Design review of the part built by this model. Coordinates are the model's own, in mm. A direction names the side the tool comes from. Give positions to 0.01 mm unless a question says otherwise; leave off trailing zeros. Order: outer loops, then holes, each group sorted by start corner. A loop starts at its lowest first (then second) coordinate and runs counter-clockwise, first axis right, second up. Notation, with made-up numbers: M 20.25,9.25 L 42.25,9.25 A33 ccw 42.25,37.25 Z; hole C -22,71 d6. An arc over 180 degrees is marked long. Answer as a JSON object with one key per item and string values.
from build123d import *

# Parameters (mm, degrees)
SKETCH1_W             = 152.4
SKETCH1_H             = 19.05
SKETCH1_R             = 4
BOSS_EXTRUDE1_DEPTH   = 25.4
SKETCH3_R             = 25.05
CUT_EXTRUDE1_DEPTH    = 22
M10_CLEARANCE_HOLE1_D = 11
SKETCH11_R            = 2.5
CUT_EXTRUDE2_DEPTH    = 10


with BuildPart() as part:
    # Sketch1 → Boss-Extrude1 (new body)
    with BuildSketch(Plane.XY):
        with Locations((0, -34.525)):
            Rectangle(SKETCH1_W, SKETCH1_H)
        with BuildLine():
            Line((-37.7, -25), (37.7, -25))
            Line((37.7, -25), (37.7, 0))
            ThreePointArc((37.7, 0), (0, 37.7), (-37.7, 0))
            Line((-37.7, 0), (-37.7, -25))
        make_face()
        Circle(SKETCH1_R, mode=Mode.SUBTRACT)
    extrude(amount=BOSS_EXTRUDE1_DEPTH)

    # Sketch3 → Cut-Extrude1 (cut)
    with BuildSketch(Plane.XY.offset(25.4)):
        Circle(SKETCH3_R)
    extrude(amount=-CUT_EXTRUDE1_DEPTH, mode=Mode.SUBTRACT)

    # M10 Clearance Hole1 (through all)
    with Locations(Plane(origin=(0, -25, 0), x_dir=(1, 0, 0), z_dir=(0, 1, 0))):
        with Locations((-57.2, -12.7), (57.2, -12.7)):
            Hole(M10_CLEARANCE_HOLE1_D / 2)

    # Sketch11 → Cut-Extrude2 (cut)
    with BuildSketch(Plane(origin=(0, 0, 0), x_dir=(-1, 0, 0), z_dir=(0, 0, -1))):
        with Locations((5.775120383, 13.84369837)):
            Circle(SKETCH11_R)
        with Locations((-5.705346209, 13.872599779)):
            Circle(SKETCH11_R)
        with Locations((-13.84369837, 5.775120383)):
            Circle(SKETCH11_R)
        with Locations((-13.872599779, -5.705346209)):
            Circle(SKETCH11_R)
        with Locations((-5.775120383, -13.84369837)):
            Circle(SKETCH11_R)
        with Locations((5.705346209, -13.872599779)):
            Circle(SKETCH11_R)
        with Locations((13.84369837, -5.775120383)):
            Circle(SKETCH11_R)
        with Locations((13.872599779, 5.705346209)):
            Circle(SKETCH11_R)
    extrude(amount=-CUT_EXTRUDE2_DEPTH, mode=Mode.SUBTRACT)


solid = part.part
(1) Draft analysis for pull direction Z (two halves, no side actions). For faces 1 (the flat face through (-1, -12, 0)), 2 (the cylindrical face through (-16.257, 6.456, 1.676)), 3 (the cylindrical face through (62.695, -34.658, 12.458)), 4 (the cylindrical face through (-51.705, -34.658, 12.458)), state which applies: +Z half, -Z half, draft (parallel to the pull), parting line (faces both ways), or undercut.
Checked values:
{"face 1": "-Z half", "face 2": "draft", "face 3": "undercut", "face 4": "undercut"}
(2) We need section D-D (x = 57.2). Write out the cut boundary in (y, z), plus the area to 3 significant figures.
Checked values:
{"outline": "M -44.05,0 L -25,0 L -25,7.2 L -44.05,7.2 Z; M -44.05,18.2 L -25,18.2 L -25,25.4 L -44.05,25.4 Z", "area": "274 mm^2"}
(3) We need section A-A (x = 0). Write out the cut boundary in (y, z), plus the area to 3 significant figures.
Checked values:
{"outline": "M -44.05,0 L -4,0 L -4,3.4 L -25.05,3.4 L -25.05,25.4 L -44.05,25.4 Z; M 4,0 L 37.7,0 L 37.7,25.4 L 25.05,25.4 L 25.05,3.4 L 4,3.4 Z", "area": "947 mm^2"}
(4) We need section B-B (z = 12.7). Write out the cut boundary in (x, y), plus the area to 3 significant figures.
Checked values:
{"outline": "M -76.2,-44.05 L -62.7,-44.05 L -62.7,-25 L -76.2,-25 Z; M -51.7,-44.05 L 51.7,-44.05 L 51.7,-25 L 37.7,-25 L 37.7,0 A37.7 ccw -37.7,0 L -37.7,-25 L -51.7,-25 Z; M 62.7,-44.05 L 76.2,-44.05 L 76.2,-25 L 62.7,-25 Z; hole C 0,0 d50.1", "area": "4,630 mm^2"}
(5) To check wall thickness, follow L1, parallel to Y at x = 0, z = 13; L2, parallel to Z at x = -9, y = -2; L3, parallel to X at y = 15, z = 15.5. State the ranges of each line that lie inside material, in increasing order. Write a range as from..to.
Checked values:
{"L1": "y = -44.05..-25.05, 25.05..37.7", "L2": "z = 0..3.4", "L3": "x = -34.59..-20.06, 20.06..34.59"}
(6) We need section C-C (z = 21.5). Write out the cut boundary in (x, y), plus the area to 3 significant figures.
Checked values:
{"outline": "M -76.2,-44.05 L 76.2,-44.05 L 76.2,-25 L 37.7,-25 L 37.7,0 A37.7 ccw -37.7,0 L -37.7,-25 L -76.2,-25 Z; hole C 0,0 d50.1", "area": "5,050 mm^2"}
(7) Insertion check: pin 1 (6 mm diameter, centred on x = 5.78, y = -13.84, fed in from +Z); pin 2 (4.5 mm diameter, centred on x = -13.87, y = 5.71, fed in from -Z); pin 3 (4 mm diameter, centred on y = 12.5, z = 14, fed in from +X); pin 4 (5 mm diameter, centred on x = -5.5, z = 3, fed in from +Y). Each pin has a flat end and moves straight along its axis. Give the tip position at first contact, or say it passes through.
Checked values:
{"pin 1": "stops at z = 3.4", "pin 2": "passes through", "pin 3": "stops at x = 36.21", "pin 4": "stops at y = 37.58"}
(8) Tool access review of faces 5 (the flat face through (5, 0, 3.4)), 6 (the flat face through (-37.7, -12, 13)), 7 (the cylindrical face through (-8.084, 12.886, 1.676)): name each direction out of +Z, -Z, +X, -X, +Y, -Y from which nothing blocks a thin tool from reaching the whole face with its end or side.
Checked values:
{"face 5": "+Z", "face 6": "+Z, -Z, -X, +Y", "face 7": "+Z, -Z"}
